```python
from build123d import *

# Parameters (mm, degrees)
SKETCH1_W           = 112.522
SKETCH1_H           = 66.04
SKETCH1_R           = 1.5
BOSS_EXTRUDE1_DEPTH = 3
SKETCH4_W           = 91.948
SKETCH4_H           = 44.704
BOSS_EXTRUDE2_DEPTH = 12
SHELL1_T            = -2.54
SKETCH13_R          = 3.253406585
CUT_EXTRUDE1_DEPTH  = 8.19
SKETCH15_R          = 3.393829234
CUT_EXTRUDE2_DEPTH  = 8.19
SCALE1_SCALE        = 1.5


with BuildPart() as part:
    # Sketch1 → Boss-Extrude1 (new body)
    with BuildSketch(Plane(origin=(0, 0, 0), x_dir=(1, 0, 0), z_dir=(0, 1, 0))):
        with Locations((4.991983213, -7.115654676)):
            Rectangle(SKETCH1_W, SKETCH1_H)
        with Locations(Location((-46.207741765, 20.726518927, 0), (0, 0, 270))):
            Circle(SKETCH1_R, mode=Mode.SUBTRACT)
        with Locations(Location((56.100367261, 20.726518927, 0), (0, 0, 270))):
            Circle(SKETCH1_R, mode=Mode.SUBTRACT)
        with Locations(Location((56.100367261, -35.155923699, 0), (0, 0, 270))):
            Circle(SKETCH1_R, mode=Mode.SUBTRACT)
        with Locations(Location((-46.207741765, -35.155923699, 0), (0, 0, 270))):
            Circle(SKETCH1_R, mode=Mode.SUBTRACT)
    extrude(amount=BOSS_EXTRUDE1_DEPTH)

    # Sketch4 → Boss-Extrude2 (add)
    with BuildSketch(Plane(origin=(0, 3, 0), x_dir=(1, 0, 0), z_dir=(0, 1, 0))):
        with Locations((4.991983213, -7.115654676)):
            Rectangle(SKETCH4_W, SKETCH4_H)
    extrude(amount=BOSS_EXTRUDE2_DEPTH)

    # Shell1
    shell1_openings = [part.faces().sort_by_distance(p)[0] for p in [
        (4.991983213, 15, 7.115654676),
    ]]
    offset(amount=SHELL1_T, openings=shell1_openings, kind=Kind.INTERSECTION)

    # Sketch13 → Cut-Extrude1 (cut)
    with BuildSketch(Plane.XY.offset(29.467654676)):
        with Locations((-28.892784248, 9.118527178)):
            Circle(SKETCH13_R)
    extrude(amount=-CUT_EXTRUDE1_DEPTH, mode=Mode.SUBTRACT)

    # Sketch15 → Cut-Extrude2 (cut)
    with BuildSketch(Plane.ZY.offset(40.982016787)):
        with Locations((-6.693412029, 8.197427611)):
            Circle(SKETCH15_R)
    extrude(amount=-CUT_EXTRUDE2_DEPTH, mode=Mode.SUBTRACT)


with BuildPart() as part_1:
    # Scale1: scaled about (5.236972756, 3.498136201, 7.097395086)
    add(part.part.scale(SCALE1_SCALE).moved(Location((-2.618486378, -1.7490681, -3.548697543))))


solid = part_1.part
```
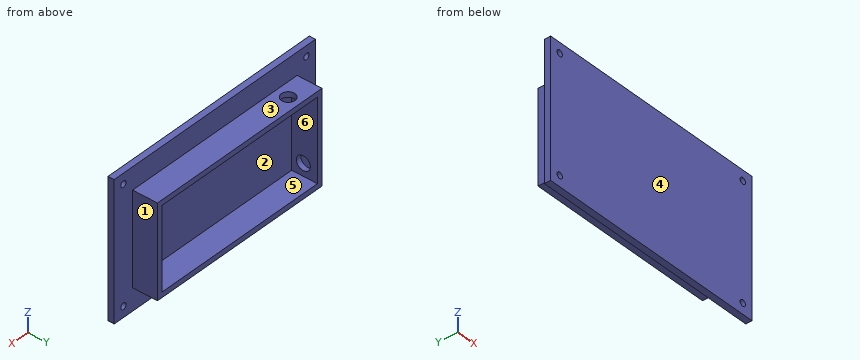
For this review, take the finished solid that the model builds, in its own axes (mm). Face numbers are marked on the shaded views. A direction names the side the tool comes from. Coordinates: 2 decimals unless noted, no trailing zeros. Loops run counter-clockwise (first coordinate to the right, second up) from the corner with the lowest first, then second, coordinate; pieces in that order, holes last. Notation, with made-up numbers: (46, 14.25) -> (94, 14.25) arc R30 cw to (94, 39.25) -> close; hole circle Ø4 at (85, -5.75). An arc over 180 degrees is marked (long way). Return JSON: item names as keys, results as strings. Group by question number.
(1) Mouldability with a two-part tool opening along Z and no side actions: class the marked faces 3, 4, 5 and 6 as pulls with the +Z half, pulls with the -Z half, needs draft (parallel to the pull), parting line crosses it, or undercut.
(2) Consider section C-C, the plane z = 42.5. Give the boundary of the cut face in (x, y).
(3) Tool access review of the marked faces 1 and 2: name each direction out of +Z, -Z, +X, -X, +Y, -Y from which nothing blocks a thin tool from reaching the whole face with its end or side.
(4) To check wall thickness, follow L1, parallel to X at y = 13, z = 32; L2, parallel to Z at x = 50, y = 7; L3, parallel to Y at x = -1, z = 32.5. State the ranges of each line that lie inside material, in increasing order.
(5) Consider section A-A, the plane x = -18. Give the boundary of the cut face in (y, z), plus the area to 3 significant figures.
(6) For pin 1 Ø9.5 at (y, z) = (11, 21) entering from +X; pin 2 Ø5 at (x, z) = (-71.93, 49.19) entering from +Y; pin 3 Ø2 at (x, z) = (3, 17) entering from +Y, all flat-tipped, find the tip position at first contact; note any pin that passes through.
(7) Consider section B-B, the plane z = 8. Give the boundary of the cut face in (x, y).
Results below:
{
 "1": {"face 3": "pulls with the +Z half", "face 4": "needs draft", "face 5": "undercut", "face 6": "undercut"},
 "2": {"outline": "(-79.52, -1.75) -> (89.26, -1.75) -> (89.26, 2.75) -> (-79.52, 2.75) -> close"},
 "3": {"face 1": "+Z, -Z, +X, +Y", "face 2": "+Y"},
 "4": {"L1": "x = -64.09 to -60.28, 70.02 to 73.83", "L2": "z = -26.4 to -22.59, 36.84 to 40.65", "L3": "y = -1.75 to 2.06"},
 "5": {"outline": "(-1.75, -42.41) -> (2.75, -42.41) -> (2.75, -26.4) -> (20.75, -26.4) -> (20.75, -22.59) -> (2.06, -22.59) -> (2.06, 36.84) -> (20.75, 36.84) -> (20.75, 40.65) -> (2.75, 40.65) -> (2.75, 56.65) -> (-1.75, 56.65) -> close", "area": "542 mm2"},
 "6": {"pin 1": "stops at x = 73.83", "pin 2": "stops at y = 2.75", "pin 3": "stops at y = 2.06"},
 "7": {"outline": "(-79.52, -1.75) -> (89.26, -1.75) -> (89.26, 2.75) -> (73.83, 2.75) -> (73.83, 20.75) -> (70.02, 20.75) -> (70.02, 2.06) -> (-60.28, 2.06) -> (-60.28, 20.75) -> (-64.09, 20.75) -> (-64.09, 2.75) -> (-79.52, 2.75) -> close"}
}
